For this review, use the dimensioned drawing (mm, ordinates from the lowest corner) and the shaded views. Give positions to 0.01 mm unless a question says otherwise; leave off trailing zeros. Write each loop counter-clockwise with the first axis right and the second up, starting at its lowest first coordinate (ties: lowest second). Pieces come first, ordered by that corner, then holes. Notation, with made-up numbers: (-25.5, -5.5) -> (28.5, -5.5) arc R23 cw to (28.5, 19.5) -> close; hole circle Ø6 at (-23.75, 10.25). An arc over 180 degrees is marked (long way). Return JSON: item names as keys, results as strings.
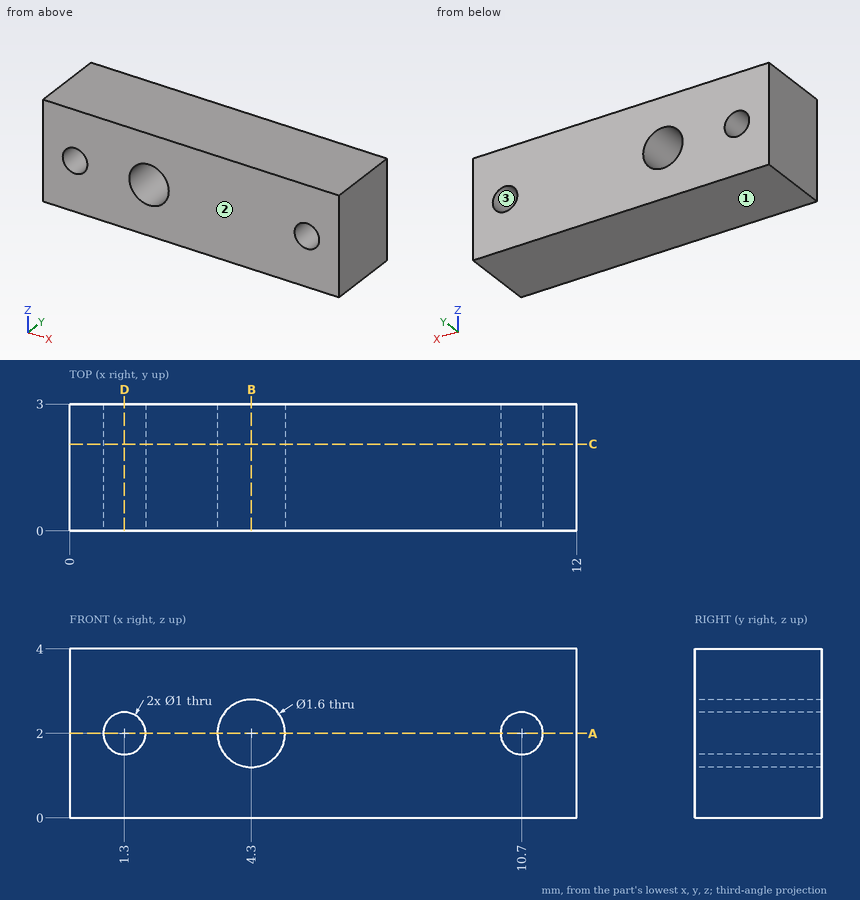
1. The part is to be moulded in two halves that separate along Z. For the marked faces 1, 2 and 3, say which applies: +Z half, -Z half, draft (parallel to the pull), parting line (faces both ways), or undercut.
Results found:
{"face 1": "-Z half", "face 2": "draft", "face 3": "undercut"}
2. Add section B-B, the plane x = 4.3. State the section outline as (y, z) points.
Results found:
{"outline": "(0, 0) -> (3, 0) -> (3, 1.2) -> (0, 1.2) -> close; (0, 2.8) -> (3, 2.8) -> (3, 4) -> (0, 4) -> close"}
3. Add section A-A, the plane z = 2. State the section outline as (x, y) points.
Results found:
{"outline": "(0, 0) -> (0.8, 0) -> (0.8, 3) -> (0, 3) -> close; (1.8, 0) -> (3.5, 0) -> (3.5, 3) -> (1.8, 3) -> close; (5.1, 0) -> (10.2, 0) -> (10.2, 3) -> (5.1, 3) -> close; (11.2, 0) -> (12, 0) -> (12, 3) -> (11.2, 3) -> close"}
4. Add section D-D, the plane x = 1.3. State the section outline as (y, z) points, plus the area to 3 significant figures.
Results found:
{"outline": "(0, 0) -> (3, 0) -> (3, 1.5) -> (0, 1.5) -> close; (0, 2.5) -> (3, 2.5) -> (3, 4) -> (0, 4) -> close", "area": "9.00 mm²"}
5. To check wall thickness, follow probe 1 along X at (y, z) = (0.95, 2); probe 2 along Z at (x, y) = (10.7, 2.05); probe 3 along Z at (x, y) = (4.3, 1.5). State the ranges of each line that lie inside material, in increasing order.
Results found:
{"probe 1": "x = 0 to 0.8, 1.8 to 3.5, 5.1 to 10.2, 11.2 to 12", "probe 2": "z = 0 to 1.5, 2.5 to 4", "probe 3": "z = 0 to 1.2, 2.8 to 4"}
6. Add section C-C, the plane y = 2.05. State the section outline as (x, z) points.
Results found:
{"outline": "(0, 0) -> (12, 0) -> (12, 4) -> (0, 4) -> close; hole circle Ø1 at (1.3, 2); hole circle Ø1.6 at (4.3, 2); hole circle Ø1 at (10.7, 2)"}
